```python
from build123d import *

# Parameters (mm, degrees)
SKETCH019_R             = 1.130326
PAD016_DEPTH            = 1
SKETCH020_W             = 5.904956
SKETCH020_H             = 7.129152
SKETCH020_W_2           = 14.33032
SKETCH020_H_2           = 9.073469
SKETCH020_W_3           = 13.041881
SKETCH020_H_3           = 7.469439
SKETCH020_W_4           = 2.541733
SKETCH020_H_4           = 6.479892
PAD017_DEPTH            = 1
PAD017_FACE36_W         = 7.129152
PAD017_FACE36_H         = 5.904956
PAD018_DEPTH            = 6.2
PAD018_FACE35_W         = 9.073469
PAD018_FACE35_H         = 14.33032
PAD019_DEPTH            = 10
PAD019_FACE34_W         = 7.469439
PAD019_FACE34_H         = 13.041881
PAD020_DEPTH            = 3.5
POCKET003_DEPTH         = 11
SKETCH022_R             = 1.91
PAD021_DEPTH            = 3.5
SKETCH023_R             = 2.22864
SKETCH023_R_2           = 1.768375
PAD022_DEPTH            = 2
BODY003_ROLL_ANGLE      = 180
BODY003_PLACEMENT_ANGLE = 90


with BuildPart() as part:
    # Sketch019 → Pad016 (new body)
    with BuildSketch(Plane.XY):
        Polygon((-15.284975, 18.270082), (-14.928669, -5.910554), (-13.97018, -7.070244), (4.600039, -7.070244), (9.354287, -2.482894), (9.354287, 20.950066), (8.622145, 21.624855), (5.667069, 21.624855), (5.667069, 29.864458), (4.754071, 30.908138), (-3.262787, 30.908138), align=None)
        with Locations((-13.437825, 16.870399)):
            Circle(SKETCH019_R, mode=Mode.SUBTRACT)
        with Locations((-13.075155, -4.675778)):
            Circle(SKETCH019_R, mode=Mode.SUBTRACT)
        with Locations((4.913836, -2.591921)):
            Circle(SKETCH019_R, mode=Mode.SUBTRACT)
    extrude(amount=PAD016_DEPTH)

    # Sketch020 (on Face16 of Pad016) → Pad017 (join)
    with BuildSketch(Plane.XY.offset(1)):
        with Locations((2.196002, 26.239064)):
            Rectangle(SKETCH020_W, SKETCH020_H)
        with Locations((2.159996, 15.4733225)):
            Rectangle(SKETCH020_W_2, SKETCH020_H_2)
        with Locations((2.0113995, 5.2073215)):
            Rectangle(SKETCH020_W_3, SKETCH020_H_3)
        with Locations((-13.1164825, 3.486279)):
            Rectangle(SKETCH020_W_4, SKETCH020_H_4)
    extrude(amount=PAD017_DEPTH)

    # Pad017 Face36 → Pad018 (add)
    with BuildSketch(Plane(origin=(2.196002, 26.239064, 2), x_dir=(0, 1, 0), z_dir=(0, 0, 1))):
        Rectangle(PAD017_FACE36_W, PAD017_FACE36_H)
    extrude(amount=PAD018_DEPTH)

    # Pad018 Face35 → Pad019 (add)
    with BuildSketch(Plane(origin=(2.159996, 15.4733225, 2), x_dir=(0, 1, 0), z_dir=(0, 0, 1))):
        Rectangle(PAD018_FACE35_W, PAD018_FACE35_H)
    extrude(amount=PAD019_DEPTH)

    # Pad019 Face34 → Pad020 (add)
    with BuildSketch(Plane(origin=(2.0113995, 5.2073215, 2), x_dir=(0, 1, 0), z_dir=(0, 0, 1))):
        Rectangle(PAD019_FACE34_W, PAD019_FACE34_H)
    extrude(amount=PAD020_DEPTH)

    # Sketch021 (on Face38 of Pad020) → Pocket003 (cut)
    with BuildSketch(Plane(origin=(-5.005164, 0, 0), x_dir=(0, -1, 0), z_dir=(-1, 0, 0))):
        with BuildLine():
            ThreePointArc((-10.909353, 7.32661), (-15.4381290695, 12.0450982539), (-20.065739, 7.4235))
            Line((-20.065739, 7.4235), (-23.086145, 11.442731))
            Line((-23.086145, 11.442731), (-16.489733, 15.336999))
            Line((-16.489733, 15.336999), (-4.992367, 12.502396))
            Line((-4.992367, 12.502396), (-10.909353, 7.32661))
        make_face()
    extrude(amount=-POCKET003_DEPTH, mode=Mode.SUBTRACT)

    # Sketch022 (on Face44 of Pocket003) → Pad021 (join)
    with BuildSketch(Plane.YZ.offset(5.14848)):
        with Locations((26.402317, 5.299071)):
            Circle(SKETCH022_R)
    extrude(amount=PAD021_DEPTH)

    # Sketch023 (on Face36 of Pad021) → Pad022 (join)
    with BuildSketch(Plane.YZ.offset(8.53234)):
        with Locations((5.306993, 3.250137)):
            Circle(SKETCH023_R)
        with Locations((5.306993, 3.250137)):
            Circle(SKETCH023_R_2, mode=Mode.SUBTRACT)
    extrude(amount=PAD022_DEPTH)


with BuildPart() as part_1:
    # Body003 roll: moved
    add(part.part.rotate(Axis((0, 0, 0), (1, 0, 0)), BODY003_ROLL_ANGLE))


with BuildPart() as part_2:
    # Body003 placement: moved
    add(part_1.part.moved(Location((18.8, 4.5, -4.4))).rotate(Axis((18.8, 4.5, -4.4), (0, 0, 1)), BODY003_PLACEMENT_ANGLE))


solid = part_2.part
```
The model under review builds one solid part; all positions refer to its coordinate system, in mm. A direction names the side the tool comes from. Give positions to 0.01 mm unless a question says otherwise; leave off trailing zeros. Write each loop counter-clockwise with the first axis right and the second up, starting at its lowest first coordinate (ties: lowest second). Pieces come first, ordered by that corner, then holes. Notation, with made-up numbers: M 35,-19 L 59,-19 A20 ccw 59,1 Z; hole C 15.5,70 d8. An arc over 180 degrees is marked long. Write each question's results on one line, items separated by ' | '. Start each with the question number.
1. We need section B-B (z = -13.25). Write out the cut boundary in (x, y).
2. Mouldability with a two-part tool opening along X and no side actions: class faces 4 (the flat face through (20.273, 7, -8)), 5 (the flat face through (45, 3.744, -9)), 6 (the flat face through (41.474, 7, -9)) as released by +X, released by -X, zero draft, split by the parting line, or undercut.
3. We need section C-C (x = 25). Write out the cut boundary in (y, z).
4. We need section A-A (y = 5). Write out the cut boundary in (x, z).
5. For faces 1 (the flat face through (38, 10.495, -15)), 2 (the flat face through (28, 13.854, -5)), 3 (the flat face through (29.737, 7, -10)), list the 3-axis set-ups (+Z, -Z, +X, -X, +Y, -Y) from which the entire face can be reached by the end or side of a thin tool; tool diameter is ignored.
6. For probe 1 along X at (y, z) = (12.5, -9.75); probe 2 along X at (y, z) = (6.5, -6.5); probe 3 along X at (y, z) = (4.75, -11.75), list the stretches that pass through material, from the lowest coordinate up. Write a range as [from, to].
7. We need section D-D (x = 45). Write out the cut boundary in (y, z).
8. Insertion check: pin 1 Ø6 at (x, y) = (25, 5.5) entering from -Z; pin 2 Ø2 at (x, z) = (45, -7.5) entering from -Y; pin 3 Ø0.5 at (y, z) = (-8.5, -6) entering from -X; pin 4 Ø1 at (y, z) = (-6, -7) entering from -X. Each pin has a flat end and moves straight along its axis. Give the tip position at first contact, or say it passes through.
Results found:
1) outline: M 29.74,10.49 L 29.92,10.49 L 29.92,-0.51 L 38.65,-0.51 L 38.65,10.49 L 38.81,10.49 L 38.81,13.83 L 29.74,13.83 Z
2) face 4: released by -X | face 5: zero draft | face 6: undercut
3) outline: M -10.61,-5.4 L -9.89,-5.4 L -9.89,-6.4 L -7.35,-6.4 L -7.35,-5.4 L -0.01,-5.4 L -0.01,-9.9 L 13.03,-9.9 L 13.03,-9.69 L 15.03,-9.69 L 15.03,-9.18 L 13.03,-9.18 L 13.03,-6.12 L 15.03,-6.12 L 15.03,-5.61 L 13.03,-5.61 L 13.03,-5.4 L 13.85,-5.4 L 13.85,-4.4 L -10.61,-4.4 Z
4) outline: M 11.73,-5.4 L 20.27,-5.4 L 20.27,-9.9 L 27.74,-9.9 L 27.74,-5.4 L 29.74,-5.4 L 29.74,-12.38 A4.58 ccw 33.64,-16.4 L 34.93,-16.4 A4.58 ccw 38.81,-12.58 L 38.81,-5.4 L 41.47,-5.4 L 41.47,-12.6 L 48.6,-12.6 L 48.6,-5.4 L 49.71,-5.4 L 49.71,-4.4 L 11.73,-4.4 Z
5) face 1: -Z, +X, -Y | face 2: +Z, +X, -X, +Y | face 3: -Z, +Y, -Y
6) probe 1: x = [20.27, 27.74], [29.74, 38.81], [43.29, 47.11] | probe 2: x = [20.27, 27.74], [29.74, 38.81], [41.47, 48.6] | probe 3: x = [29.74, 38.81], [41.47, 48.6]
7) outline: M -3.24,-5.4 L 3.74,-5.4 L 3.74,-12.6 L 9.65,-12.6 L 9.65,-11.6 L 13.15,-11.6 L 13.15,-7.8 L 9.65,-7.8 L 9.65,-5.4 L 10.17,-5.4 L 10.17,-4.4 L -3.24,-4.4 Z
8) pin 1: stops at z = -9.9 | pin 2: stops at y = 3.74 | pin 3: stops at x = 19.05 | pin 4: passes through
